Build history of the part. All positions in model axes, mm. A direction names the side the tool comes from. Round coordinates to 2 decimals unless told otherwise and drop trailing zeros. Write each loop counter-clockwise with the first axis right and the second up, starting at its lowest first coordinate (ties: lowest second). Pieces come first, ordered by that corner, then holes. Notation, with made-up numbers: M 77.25,54 L 120.25,54 A22 cw 120.25,65 Z; hole C -16,-19 d7. An arc over 180 degrees is marked long. Use a Markdown table: item, result.
from build123d import *

# Parameters (mm, degrees)
SKETCH1_W           = 14.417582417
SKETCH1_H           = 150
SKETCH2_R           = 29.538461538
BOSS_EXTRUDE1_DEPTH = 20


with BuildPart() as part:
    # Sketch1 → Revolve1 (revolve)
    with BuildSketch(Plane.XY):
        with Locations((22.32967033, 41.065934066)):
            Rectangle(SKETCH1_W, SKETCH1_H)
    revolve(axis=Axis((0, 46.065934066, 0), (0, -1, 0)))

    # Sketch2 → Boss-Extrude1 (add)
    with BuildSketch(Plane.XY):
        with Locations((0, 116.065934066)):
            Circle(SKETCH2_R)
        with Locations((0, -33.934065934)):
            Circle(SKETCH2_R)
    extrude(amount=BOSS_EXTRUDE1_DEPTH)


solid = part.part
Q1. Cut at B-B on z = -5.5. Give the cut face in (x, y).
Response values:
| item | result |
|---|---|
| outline | M -29.02,-33.93 L -14.09,-33.93 L -14.09,116.07 L -29.02,116.07 Z; M 14.09,-33.93 L 29.02,-33.93 L 29.02,116.07 L 14.09,116.07 Z |
Q2. Cut at A-A on x = 0. Give the cut face in (y, z), and give its area (3 significant figures).
Response values:
| item | result |
|---|---|
| outline | M -63.47,0 L -4.4,0 L -4.4,15.12 L 86.53,15.12 L 86.53,0 L 145.6,0 L 145.6,20 L 116.07,20 L 116.07,29.54 L -33.93,29.54 L -33.93,20 L -63.47,20 Z; M -33.93,-29.54 L 116.07,-29.54 L 116.07,-15.12 L -33.93,-15.12 Z |
| area | 6,400 mm2 |
Q3. Drill centre lines: L1, parallel to Z at x = -0.5, y = 67; L2, parallel to Z at x = -3, y = 84; L3, parallel to Y at x = 17, z = -11.5. Where is each one in solid material? Low to high.
Response values:
| item | result |
|---|---|
| L1 | z = -29.53 to -15.11, 15.11 to 29.53 |
| L2 | z = -29.39 to -14.82, 14.82 to 29.39 |
| L3 | y = -33.93 to 116.07 |
Q4. Cut at C-C on y = 101. Give the cut face in (x, z), and give its area (3 significant figures).
Response values:
| item | result |
|---|---|
| outline | M -25.41,15.07 A29.54 ccw long 25.41,15.07 L 25.41,20 L 21.74,20 A29.54 ccw -21.74,20 L -25.41,20 Z; hole M -15.12,0 A15.12 ccw 15.12,0 Z |
| area | 2,400 mm2 |
Q5. Which spindle directions (+Z, -Z, +X, -X, +Y, -Y) get a long thin tool onto all of the face, cutting with end or side? Do faces 5 (the flat face through (0, -33.934, 24)), 6 (the cylindrical face through (0.222, -4.396, 5.774)), 7 (the flat face through (0, -34, 0)), 8 (the flat face through (0, 116, 0)). Say none if no direction does.
Response values:
| item | result |
|---|---|
| face 5 | +Z, +X, -X, -Y |
| face 6 | none |
| face 7 | -Y |
| face 8 | +Y |
Q6. Drop flat-ended pins along their axis: P1, Ø1, axis at x = 7.5, y = 89.5, coming from the -Z side; P2, Ø8, axis at x = 8.5, y = 21.5, coming from the -Z side; P3, Ø24, axis at x = 0, z = 0, coming from the -Y side. Give the stop position or say it passes through.
Response values:
| item | result |
|---|---|
| P1 | stops at z = -28.7 |
| P2 | stops at z = -29.19 |
| P3 | stops at y = -63.47 |
Q7. Two-plate mould, pull along Y, no slides. Class faces 1 (the flat face through (0, -33.934, -18)), 2 (the flat face through (0, 116.066, 24)), 3 (the flat face through (0, -44, 20)), 4 (the cylindrical face through (-3.28, 42.12, -14.76)): +Y half, -Y half, draft (parallel to the pull), parting line (faces both ways), or undercut.
Response values:
| item | result |
|---|---|
| face 1 | -Y half |
| face 2 | +Y half |
| face 3 | draft |
| face 4 | undercut |
Q8. Cut at D-D on x = -10.5. Give the cut face in (y, z).
Response values:
| item | result |
|---|---|
| outline | M -61.54,0 L -6.32,0 L -6.32,10.88 L 88.46,10.88 L 88.46,0 L 143.68,0 L 143.68,20 L 116.07,20 L 116.07,27.61 L -33.93,27.61 L -33.93,20 L -61.54,20 Z; M -33.93,-27.61 L 116.07,-27.61 L 116.07,-10.88 L -33.93,-10.88 Z |
